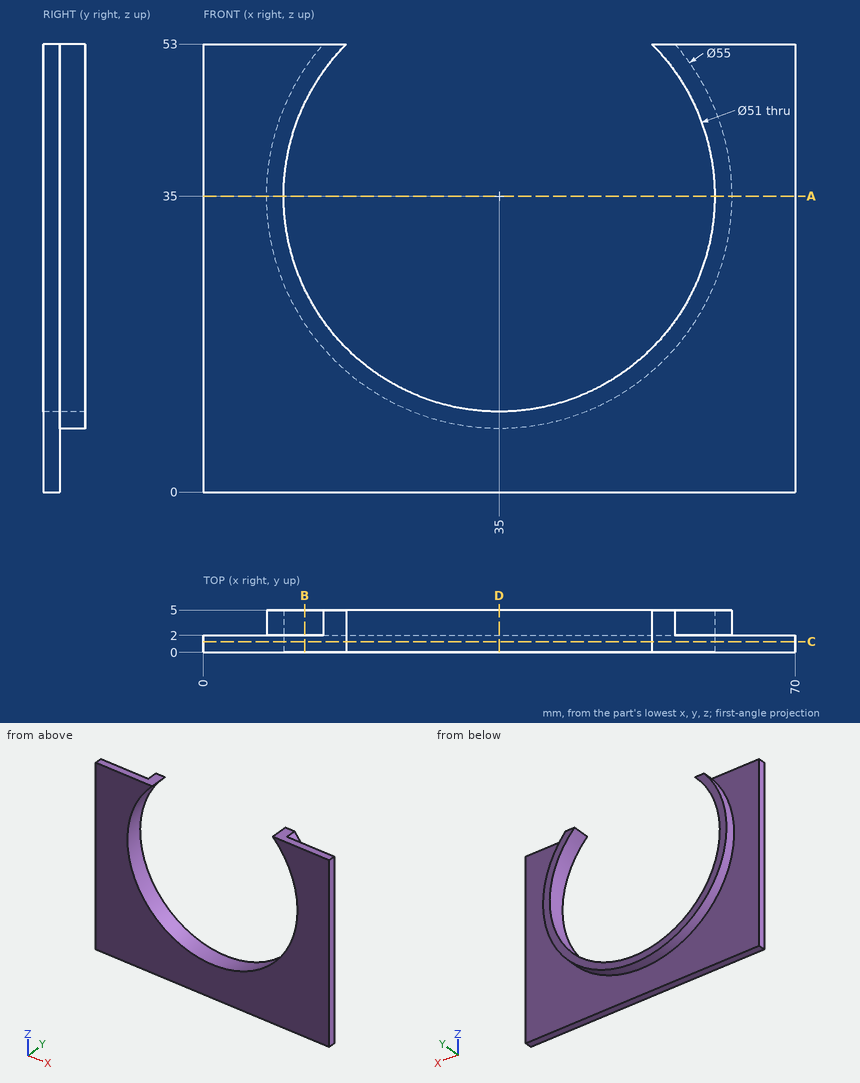
Here's the drawing with two shaded views (mm, measured from the low corner). I have some questions. Give positions to 0.01 mm unless a question says otherwise; leave off trailing zeros. Write each loop counter-clockwise with the first axis right and the second up, starting at its lowest first coordinate (ties: lowest second). Pieces come first, ordered by that corner, then holes. Notation, with made-up numbers: (-22, 19) -> (37, 19) arc R9 cw to (37, 27) -> close; hole circle Ø7 at (-1.75, 25.5). An arc over 180 degrees is marked (long way). One line per item, written item: value.
Q1. For P1, Ø5, axis at x = 63, z = 17.5, coming from the +Y side, with a flat end and sliding along its axis, tell me the tip position at first contact or that it passes through.
Results found:
P1: stops at y = 2
Q2. Please list where these lines run through material, in increasing order: line 1 (X direction, y = 1.3, z = 35); line 2 (X direction, y = 1.55, z = 39); line 3 (Z direction, x = 35, y = 3.15). Write a range as [from, to].
Results found:
line 1: x = [0, 9.5], [60.5, 70]
line 2: x = [0, 9.82], [60.18, 70]
line 3: z = [7.5, 9.5]
Q3. Imagine slicing it at A-A on z = 35. Please give me the cut outline in (x, y).
Results found:
outline: (0, 0) -> (9.5, 0) -> (9.5, 5) -> (7.5, 5) -> (7.5, 2) -> (0, 2) -> close; (60.5, 0) -> (70, 0) -> (70, 2) -> (62.5, 2) -> (62.5, 5) -> (60.5, 5) -> close
Q4. Imagine slicing it at D-D on x = 35. Please give me the cut outline in (y, z).
Results found:
outline: (0, 0) -> (2, 0) -> (2, 7.5) -> (5, 7.5) -> (5, 9.5) -> (0, 9.5) -> close
Q5. Imagine slicing it at B-B on x = 12. Please give me the cut outline in (y, z), and give its area (3 significant figures).
Results found:
outline: (0, 0) -> (2, 0) -> (2, 19.93) -> (5, 19.93) -> (5, 23.99) -> (0, 23.99) -> close; (0, 46.01) -> (5, 46.01) -> (5, 50.07) -> (2, 50.07) -> (2, 53) -> (0, 53) -> close
area: 86.3 mm^2
Q6. Imagine slicing it at C-C on y = 1.25. Please give me the cut outline in (x, z).
Results found:
outline: (0, 0) -> (70, 0) -> (70, 53) -> (53.06, 53) arc R25.5 cw (long way) to (16.94, 53) -> (0, 53) -> close
